Could you check a few things on this model? Use its own coordinates, in mm. Face numbers are marked on the shaded views. A direction names the side the tool comes from. Coordinates: 2 decimals unless noted, no trailing zeros. Loops run counter-clockwise (first coordinate to the right, second up) from the corner with the lowest first, then second, coordinate; pieces in that order, holes last.
1) Will these pins go through, and if not, where does the flat tip stop? P1, Ø3.5, axis at x = -23, z = 10, coming from the +Y side; P2, Ø10, axis at x = 23, z = 10, coming from the +Y side; P3, Ø4, axis at y = 21.5, z = 10.5, coming from the -X side.
2) If I drill on line 1 along Y through (x, z) = (-23, 4); line 2 along X through (y, z) = (-9.25, 2.75); line 3 along Y through (x, z) = (-23, 15), over which ranges is the centre line in solid material (lowest first)?
3) Imagine slicing it at C-C on y = -10. Please give me the cut outline in (x, z), plus the area to 3 significant figures.
4) Thinking about a two-plate mould opening in X: for the marked faces 3, 4, 5 and 6, which applies, released by +X, released by -X, zero draft, split by the parting line, or undercut?
5) Imagine slicing it at A-A on x = -23. Give the number of separate pieces and of enclosed holes in the cut face, plus the area to 3 significant figures.
6) Imagine slicing it at B-B on x = 0. Please give me the cut outline in (y, z), plus the area to 3 significant figures.
7) For the marked faces 1 and 2, which set-ups out of +Z, -Z, +X, -X, +Y, -Y let a thin tool reach every point of the face, with its end or its side?
8) Imagine slicing it at D-D on y = 14. Please give me the cut outline in (x, z), plus the area to 3 significant figures.
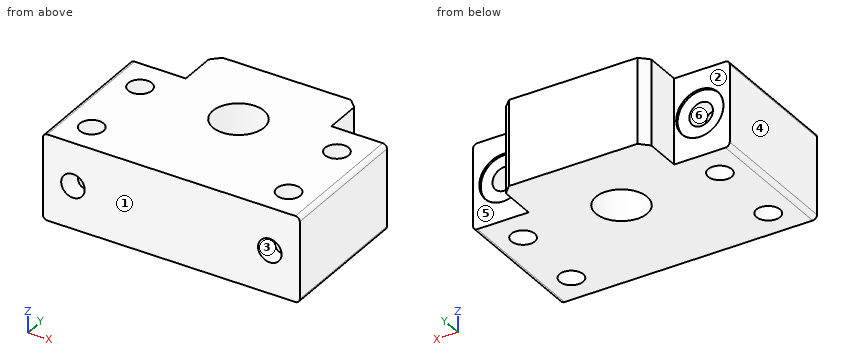
```python
from build123d import *

# Parameters (mm, degrees)
SKETCH_1_R                  = 6
SKETCH_1_R_2                = 2.75
EXTRUDE_1_DEPTH             = 20
CHAMFER_1_SIZE              = 2
FILLET_1_R                  = 1
HOLE_WIZARD_M5_1_AT_2_COUNT = 2
HOLE_WIZARD_M5_1_AT_2_PITCH = 46


with BuildPart() as part:
    # 草图1 → 凸台-拉伸1 (new body)
    with BuildSketch(Plane.XY):
        Polygon((-17, 16.25), (-17, 26.75), (17, 26.75), (17, 16.25), (30, 16.25), (30, -16.25), (-30, -16.25), (-30, 16.25), align=None)
        with Locations((0, 8.75)):
            Circle(SKETCH_1_R, mode=Mode.SUBTRACT)
        with Locations((-23, 8.75)):
            Circle(SKETCH_1_R_2, mode=Mode.SUBTRACT)
        with Locations((-23, -9.25)):
            Circle(SKETCH_1_R_2, mode=Mode.SUBTRACT)
        with Locations((23, -9.25)):
            Circle(SKETCH_1_R_2, mode=Mode.SUBTRACT)
        with Locations((23, 8.75)):
            Circle(SKETCH_1_R_2, mode=Mode.SUBTRACT)
    extrude(amount=EXTRUDE_1_DEPTH)

    # 倒角1
    chamfer_1_edges = [part.edges().sort_by_distance(p)[0] for p in [
        (-17, 26.75, 10),
        (17, 26.75, 10),
    ]]
    chamfer(chamfer_1_edges, length=CHAMFER_1_SIZE)

    # 圆角1
    fillet_1_edges = [part.edges().sort_by_distance(p)[0] for p in [
        (30, 0, 0),
        (-30, 0, 20),
        (30, 0, 20),
        (-30, 0, 0),
    ]]
    fillet(fillet_1_edges, radius=FILLET_1_R)

    # 草图3 → M5 六角头螺栓的柱形沉头孔1 (revolve, cut)
    with BuildSketch(Plane(origin=(23, 16.25, 10), x_dir=(0, 0, 1), z_dir=(1, 0, 0))):
        Polygon((0, 0), (0, 32.5), (2.75, 32.5), (2.75, 0.5), (5.5, 0.5), (5.5, 0.025), (5.525, 0), align=None)
    hole_wizard_m5_1 = revolve(axis=Axis((23, 22.6, 10), (0, -1, 0)), mode=Mode.SUBTRACT)

    # M5 六角头螺栓的柱形沉头孔1 at 2: M5 六角头螺栓的柱形沉头孔1 ×2
    with Locations(*[(-i * HOLE_WIZARD_M5_1_AT_2_PITCH, 0, 0) for i in range(1, HOLE_WIZARD_M5_1_AT_2_COUNT)]):
        add(hole_wizard_m5_1, mode=Mode.SUBTRACT)


solid = part.part
```
Filled in:
1. P1: passes through
1. P2: stops at y = 15.75
1. P3: stops at x = -17
2. line 1: y = -16.25 to -12, -6.5 to 6, 11.5 to 16.25
2. line 2: x = -30 to -25.75, -20.25 to 20.25, 25.75 to 30
2. line 3: y = -16.25 to -12, -6.5 to 6, 11.5 to 15.75
3. outline: (-30, 1) arc R1 ccw to (-29, 0) - (-25.65, 0) - (-25.65, 9.25) arc R2.75 cw to (-25.65, 10.75) - (-25.65, 20) - (-29, 20) arc R1 ccw to (-30, 19) - close; (-20.35, 0) - (20.35, 0) - (20.35, 9.25) arc R2.75 cw to (20.35, 10.75) - (20.35, 20) - (-20.35, 20) - (-20.35, 10.75) arc R2.75 cw to (-20.35, 9.25) - close; (25.65, 0) - (29, 0) arc R1 ccw to (30, 1) - (30, 19) arc R1 ccw to (29, 20) - (25.65, 20) - (25.65, 10.75) arc R2.75 cw to (25.65, 9.25) - close
3. area: 987 mm2
4. face 3: undercut
4. face 4: released by -X
4. face 5: zero draft
4. face 6: undercut
5. separate pieces: 6
5. enclosed holes: 0
5. area: 309 mm2
6. outline: (-16.25, 0) - (2.75, 0) - (2.75, 20) - (-16.25, 20) - close; (14.75, 0) - (26.75, 0) - (26.75, 20) - (14.75, 20) - close
6. area: 620 mm2
7. face 1: +Z, -Z, +X, -X, -Y
7. face 2: +Z, -Z, -X, +Y
8. outline: (-30, 1) arc R1 ccw to (-29, 0) - (-2.9, 0) - (-2.9, 20) - (-29, 20) arc R1 ccw to (-30, 19) - close; (2.9, 0) - (29, 0) arc R1 ccw to (30, 1) - (30, 19) arc R1 ccw to (29, 20) - (2.9, 20) - close; hole circle Ø5.5 at (-23, 10); hole circle Ø5.5 at (23, 10)
8. area: 1,040 mm2
